```python
from build123d import *

# Parameters (mm, degrees)
F0_R     = 8
F0_R_2   = 4
F1_DEPTH = 12
F3_R     = 12
F4_DEPTH = 4


with BuildPart() as f1:
    # F0 (on Top) → F1 (new body)
    with BuildSketch(Plane.XY):
        Circle(F0_R)
        Circle(F0_R_2, mode=Mode.SUBTRACT)
    extrude(amount=F1_DEPTH)

    # F3 (on offset) → F4 (join)
    with BuildSketch(Plane.XY.offset(12)):
        Circle(F3_R)
    extrude(amount=F4_DEPTH)


solid = f1.part
```
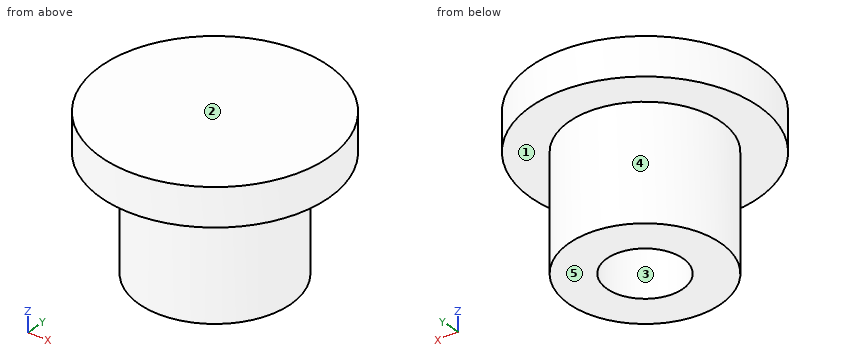
Model file for the job. Use its own axes, mm. Face numbers are marked on the shaded views. A direction names the side the tool comes from. Round coordinates to 2 decimals unless told otherwise and drop trailing zeros. Write each loop counter-clockwise with the first axis right and the second up, starting at its lowest first coordinate (ties: lowest second). Pieces come first, ordered by that corner, then holes. Notation, with made-up numbers: (-4, 17) - (48, 17) arc R16 cw to (48, 25) - close; hole circle Ø10 at (2.25, 47). An arc over 180 degrees is marked (long way). One line per item, written item: value.
(1) Cut at C-C, the plane z = 7. Give the cut face in (x, y).
Values follow:
outline: circle Ø16 at (0, 0); hole circle Ø8 at (0, 0)
(2) Two-plate mould, pull along X, no slides. Class the marked faces 3, 4 and 5: pulls with the +X half, pulls with the -X half, needs draft (parallel to the pull), parting line crosses it, or undercut.
Values follow:
face 3: undercut
face 4: parting line crosses it
face 5: needs draft
(3) Cut at A-A, the plane x = 0. Give the cut face in (y, z), plus the area to 3 significant figures.
Values follow:
outline: (-12, 12) - (-8, 12) - (-8, 0) - (-4, 0) - (-4, 12) - (4, 12) - (4, 0) - (8, 0) - (8, 12) - (12, 12) - (12, 16) - (-12, 16) - close
area: 192 mm²
(4) Cut at D-D, the plane z = 15. Give the cut face in (x, y), plus the area to 3 significant figures.
Values follow:
outline: circle Ø24 at (0, 0)
area: 452 mm²
(5) 3-axis set-ups, long thin cutter, end or side, ignore diameter. For the marked faces 1 and 2: which of +Z, -Z, +X, -X, +Y, -Y reach the whole face in a straight line?
Values follow:
face 1: -Z
face 2: +Z, +X, -X, +Y, -Y
(6) Wall check: probe 1 along Y at (x, z) = (0, 7.75); probe 2 along Z at (x, y) = (4.25, -7); probe 3 along X at (y, z) = (0.75, 3). Give the ranges that are in metal, low to high.
Values follow:
probe 1: y = -8 to -4, 4 to 8
probe 2: z = 12 to 16
probe 3: x = -7.96 to -3.93, 3.93 to 7.96
(7) Drop flat-ended pins along their axis: P1, Ø1.5, axis at y = 7, z = 5, coming from the +X side; P2, Ø4, axis at x = 1, y = 1.5, coming from the -Z side; P3, Ø8, axis at y = -4.5, z = 12.5, coming from the +X side. Give the stop position or say it passes through.
Values follow:
P1: stops at x = 4.99
P2: stops at z = 12
P3: stops at x = 11.99
